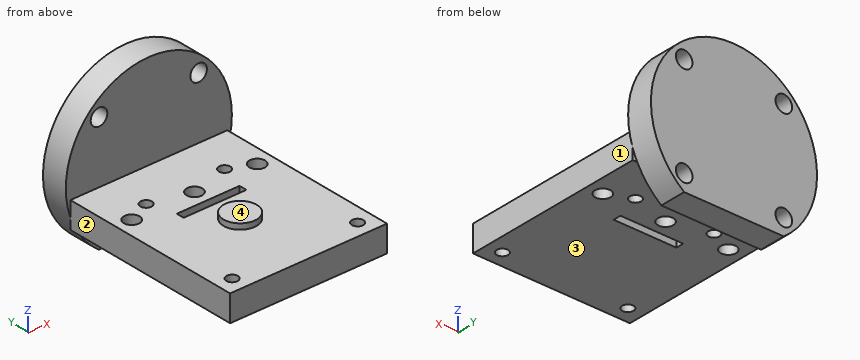
```python
from build123d import *

# Parameters (mm, degrees)
SKETCH1_R            = 1.5875
BOSS_EXTRUDE3_DEPTH  = 5
SKETCH2_R            = 1.5875
BOSS_EXTRUDE4_DEPTH  = 5
BOSS_EXTRUDE9_START  = -2.245
SKETCH3_W            = 30
SKETCH3_H            = 35
SKETCH3_R            = 1.0922
SKETCH3_R_2          = 3.175
SKETCH3_W_2          = 12
SKETCH3_H_2          = 1.5
BOSS_EXTRUDE9_DEPTH  = 5
SKETCH11_R           = 3.175
BOSS_EXTRUDE10_DEPTH = 6.07
SKETCH12_R           = 1.5
CUT_EXTRUDE2_DEPTH   = 5


with BuildPart() as part:
    # Sketch1 → Boss-Extrude3 (new body)
    with BuildSketch(Plane(origin=(0, 0, 0), x_dir=(1, 0, 0), z_dir=(0, 1, 0))):
        with BuildLine():
            Line((9.525, 12.7), (-9.525, 12.7))
            ThreePointArc((-9.525, 12.7), (0, -15.875), (9.525, 12.7))
        make_face()
        with Locations((-12.7, 0)):
            Circle(SKETCH1_R, mode=Mode.SUBTRACT)
        with Locations((12.7, 0)):
            Circle(SKETCH1_R, mode=Mode.SUBTRACT)
        with Locations((0, -12.7)):
            Circle(SKETCH1_R, mode=Mode.SUBTRACT)
        with Locations((9.525, 9.525)):
            Circle(SKETCH1_R, mode=Mode.SUBTRACT)
        with Locations((-9.525, 9.525)):
            Circle(SKETCH1_R, mode=Mode.SUBTRACT)
        with Locations((-9.525, -9.525)):
            Circle(SKETCH1_R, mode=Mode.SUBTRACT)
        with Locations((9.525, -9.525)):
            Circle(SKETCH1_R, mode=Mode.SUBTRACT)
    extrude(amount=BOSS_EXTRUDE3_DEPTH)

    # Sketch2 → Boss-Extrude4 (add)
    with BuildSketch(Plane(origin=(0, 0, 0), x_dir=(1, 0, 0), z_dir=(0, 1, 0))):
        with Locations((-12.7, 0)):
            Circle(SKETCH2_R)
        with Locations((0, -12.7)):
            Circle(SKETCH2_R)
        with Locations((12.7, 0)):
            Circle(SKETCH2_R)
    extrude(amount=BOSS_EXTRUDE4_DEPTH)

    # Sketch3 → Boss-Extrude9 (add)
    with BuildSketch(Plane.XY.offset(BOSS_EXTRUDE9_START)):
        with Locations((0, -17.5)):
            Rectangle(SKETCH3_W, SKETCH3_H)
        with Locations((-7.5, -8)):
            Circle(SKETCH3_R, mode=Mode.SUBTRACT)
        with Locations((7.5, -8)):
            Circle(SKETCH3_R, mode=Mode.SUBTRACT)
        with Locations((0, -20)):
            Circle(SKETCH3_R_2, mode=Mode.SUBTRACT)
        with Locations((-12, -32)):
            Circle(SKETCH3_R, mode=Mode.SUBTRACT)
        with Locations((12, -32)):
            Circle(SKETCH3_R, mode=Mode.SUBTRACT)
        with Locations((0, -13.75)):
            Rectangle(SKETCH3_W_2, SKETCH3_H_2, mode=Mode.SUBTRACT)
    extrude(amount=-BOSS_EXTRUDE9_DEPTH)

    # Sketch11 → Boss-Extrude10 (add)
    with BuildSketch(Plane(origin=(0, 0, -7.245), x_dir=(-1, 0, 0), z_dir=(0, 0, -1))):
        with Locations((0, -20)):
            Circle(SKETCH11_R)
    extrude(amount=-BOSS_EXTRUDE10_DEPTH)

    # Sketch12 → Cut-Extrude2 (cut)
    with BuildSketch(Plane(origin=(0, 0, -7.245), x_dir=(-1, 0, 0), z_dir=(0, 0, -1))):
        with Locations((-12, -10)):
            Circle(SKETCH12_R)
        with Locations((0, -10)):
            Circle(SKETCH12_R)
        with Locations((12, -10)):
            Circle(SKETCH12_R)
    extrude(amount=-CUT_EXTRUDE2_DEPTH, mode=Mode.SUBTRACT)


solid = part.part
```
Source: CAD feature listing. Evaluate the final solid. Frame: model axes, mm. Face numbers are marked on the shaded views. A direction names the side the tool comes from. Give positions to 0.01 mm unless a question says otherwise; leave off trailing zeros. Loops run counter-clockwise (first coordinate to the right, second up) from the corner with the lowest first, then second, coordinate; pieces in that order, holes last. Notation, with made-up numbers: (1.5, 17.25) - (23.5, 17.25) arc R8 ccw to (23.5, 23.25) - close; hole circle Ø6 at (65, 29.5). An arc over 180 degrees is marked (long way). Use CSV: the item, a comma, the result in double quotes. Start each with the question number.
1. Section A-A (y = -8). Output: boundary loops of the cut face in (x, z) (3 decimals).
2. Section B-B (z = -8.5). Output: boundary loops of the cut face in (x, y).
3. Ray query, L1, parallel to Y at x = 12, z = -4.45; L2, parallel to Y at x = 0, z = -4.65; L3, parallel to Y at x = -9, z = 12.5. Return the intervals inside material, ascending.
4. Pin query (flat end, axial travel): pin 1 (1.6 mm diameter, centred on y = -14, z = -5.5, fed in from -X); pin 2 (4 mm diameter, centred on x = -4.5, y = -1, fed in from +Z); pin 3 (4 mm diameter, centred on x = 9.525, z = -9.525, fed in from -Y); pin 4 (3.5 mm diameter, centred on x = 9.525, z = 9.525, fed in from +Y). Return the tip coordinate at first contact, or that it passes through.
5. Section C-C (x = 12). Output: boundary loops of the cut face in (y, z) (3 decimals), then the cut area to 3 significant figures.
6. Section D-D (y = -20). Output: boundary loops of the cut face in (x, z) (3 decimals).
7. Reachability of the marked faces 1, 2, 3 and 4 from +Z, -Z, +X, -X, +Y, -Y: full face, straight path, thin tool, end or side. Return the list, or none.
Response:
1,outline,"(-15, -7.245) - (-8.592, -7.245) - (-8.592, -2.245) - (-15, -2.245) - close; (-6.408, -7.245) - (6.408, -7.245) - (6.408, -2.245) - (-6.408, -2.245) - close; (8.592, -7.245) - (15, -7.245) - (15, -2.245) - (8.592, -2.245) - close"
2,outline,"(-13.41, 0) - (-10.74, 0) - (-10.74, 5) - (-13.41, 5) - close; (-8.31, 0) - (8.31, 0) - (8.31, 5) - (-8.31, 5) - close; (10.74, 0) - (13.41, 0) - (13.41, 5) - (10.74, 5) - close"
3,L1,"-35 to -33.09, -30.91 to -11.5, -8.5 to 5"
3,L2,"-35 to -14.5, -13 to -11.5, -8.5 to 5"
3,L3,"0 to 5"
4,pin 1,"x = -15"
4,pin 2,"z = 15.63"
4,pin 3,"y = 0"
4,pin 4,"y = 5"
5,outline,"(-35, -7.245) - (-33.092, -7.245) - (-33.092, -2.245) - (-35, -2.245) - close; (-30.908, -7.245) - (-11.5, -7.245) - (-11.5, -2.245) - (-30.908, -2.245) - close; (-8.5, -7.245) - (0, -7.245) - (0, -10.393) - (5, -10.393) - (5, 10.393) - (0, 10.393) - (0, -2.245) - (-8.5, -2.245) - close"
5,area,"253 mm²"
6,outline,"(-15, -7.245) - (15, -7.245) - (15, -2.245) - (3.175, -2.245) - (3.175, -1.175) - (-3.175, -1.175) - (-3.175, -2.245) - (-15, -2.245) - close"
7,face 1,"+Z, -Z, +X, -Y"
7,face 2,"+Z, -Z, -X, -Y"
7,face 3,"-Z, +X, -X, -Y"
7,face 4,"+Z, +X, -X, -Y"
